Verification items for the finished model (mm, model axes). A direction names the side the tool comes from. Coordinates: 2 decimals unless noted, no trailing zeros. Order: outer loops, then holes, each group sorted by start corner. A loop starts at its lowest first (then second) coordinate and runs counter-clockwise, first axis right, second up. Notation, with made-up numbers: M -2.5,20.25 L 35.5,20.25 A20 ccw 35.5,59.25 Z; hole C 64,79.25 d5. An arc over 180 degrees is marked long. Return JSON: item names as keys, results as strings. Group by question number.
1. Gauge pin test, flat ends, axial feed: pin 1 (7.5 mm diameter, centred on y = 22, z = 15.5, fed in from +X); pin 2 (2 mm diameter, centred on x = 0.5, z = 27, fed in from +Y); pin 3 (7.5 mm diameter, centred on x = -10, y = -1.5, fed in from -Z). Record the tip position at first contact, or that the pin passes through.
2. Section check B-B, the plane z = 15.5. Record the cut outline in (x, y), plus the area to 3 significant figures.
3. Material ranges on line 1 along X through (y, z) = (0, 1); line 2 along Z through (x, y) = (-9, -42); line 3 along Y through (x, z) = (-21.5, -1), recorded low to high.
4. Section check D-D, the plane z = -9. Record the cut outline in (x, y).
5. Section check C-C, the plane y = -9. Record the cut outline in (x, z).
6. Section check A-A, the plane x = -12. Record the cut outline in (y, z).
7. Mould release check, pull along Y, two halves, no side actions. Record for faces 1 (the flat face through (-8, -50, 13)), 2 (the flat face through (-8, -47, -12.5)), 3 (the flat face through (-8, 45, 12)): +Y half, -Y half, draft (parallel to the pull), parting line (faces both ways), or undercut.
8. Set-up check for faces 4 (the flat face through (-15, -1, 12)), 5 (the flat face through (0, -1, 12)), 6 (the flat face through (-8, 1, 25)): record each of +Z, -Z, +X, -X, +Y, -Y from which the full face is reachable in a straight line by a thin tool's end or side.
```python
from build123d import *

# Parameters (mm, degrees)
SKIZZE1_W                       = 15
SKIZZE1_H                       = 90
AUFSATZ_LINEAR_AUSTRAGEN1_DEPTH = 25
SKIZZE2_W                       = 40
SKIZZE2_H                       = 50
AUFSATZ_LINEAR_AUSTRAGEN2_DEPTH = 5


with BuildPart() as part:
    # Skizze1 → Aufsatz-Linear austragen1 (new body)
    with BuildSketch(Plane.XY):
        with Locations((-7.5, 0)):
            Rectangle(SKIZZE1_W, SKIZZE1_H)
    extrude(amount=AUFSATZ_LINEAR_AUSTRAGEN1_DEPTH)

    # Skizze2 → Aufsatz-Linear austragen2 (add)
    with BuildSketch(Plane.XZ.offset(45)):
        with Locations((-7.5, 12.5)):
            Rectangle(SKIZZE2_W, SKIZZE2_H)
    extrude(amount=AUFSATZ_LINEAR_AUSTRAGEN2_DEPTH)


solid = part.part
```
Answers follow:
{
 "1": {"pin 1": "x = 0", "pin 2": "y = -45", "pin 3": "z = 0"},
 "2": {"outline": "M -27.5,-50 L 12.5,-50 L 12.5,-45 L 0,-45 L 0,45 L -15,45 L -15,-45 L -27.5,-45 Z", "area": "1,550 mm^2"},
 "3": {"line 1": "-15 to 0", "line 2": "0 to 25", "line 3": "-50 to -45"},
 "4": {"outline": "M -27.5,-50 L 12.5,-50 L 12.5,-45 L -27.5,-45 Z"},
 "5": {"outline": "M -15,0 L 0,0 L 0,25 L -15,25 Z"},
 "6": {"outline": "M -50,-12.5 L -45,-12.5 L -45,0 L 45,0 L 45,25 L -45,25 L -45,37.5 L -50,37.5 Z"},
 "7": {"face 1": "-Y half", "face 2": "draft", "face 3": "+Y half"},
 "8": {"face 4": "+Z, -Z, -X, +Y", "face 5": "+Z, -Z, +X, +Y", "face 6": "+Z, +X, -X, +Y"}
}
